from build123d import *

# Parameters (mm, degrees)
F0_W     = 1200
F0_H     = 500
F1_DEPTH = 250
F2_W     = 400
F2_H     = 260
F3_DEPTH = 250.001
F5_DEPTH = 250
F6_R     = 110
F7_DEPTH = 500.001
F8_R     = 180
F9_DEPTH = 500.001


with BuildPart() as f1:
    # F0 (on Front) → F1 (new body)
    with BuildSketch(Plane.XZ):
        Rectangle(F0_W, F0_H)
    extrude(amount=F1_DEPTH)

    # F2 (on face) → F3 (cut, through all)
    with BuildSketch(Plane(origin=(0, 0, 0), x_dir=(-1, 0, 0), z_dir=(0, 1, 0))):
        with Locations((-600, 0)):
            Rectangle(F2_W, F2_H)
        with Locations((600, 0)):
            Rectangle(F2_W, F2_H)
    extrude(amount=-F3_DEPTH, mode=Mode.SUBTRACT)

    # F4 (on face) → F5 (join)
    with BuildSketch(Plane.XZ.offset(250)):
        Polygon((0, 250), (-300, 0), (0, -250), (300, 0), align=None)
    extrude(amount=F5_DEPTH)

    # F6 (on face) → F7 (cut, through all)
    with BuildSketch(Plane.XZ.offset(500)):
        Circle(F6_R)
    extrude(amount=-F7_DEPTH, mode=Mode.SUBTRACT)

    # F8 (on face) → F9 (cut, through all)
    with BuildSketch(Plane(origin=(0, 0, -250), x_dir=(1, 0, 0), z_dir=(0, 0, -1))):
        Circle(F8_R)
    extrude(amount=-F9_DEPTH, mode=Mode.SUBTRACT)


solid = f1.part
Input: part model. Units: mm. Frame: model coordinates. A direction names the side the tool comes from. Coordinates: 2 decimals unless noted, no trailing zeros. Loops run counter-clockwise (first coordinate to the right, second up) from the corner with the lowest first, then second, coordinate; pieces in that order, holes last.
(1) Pull-direction query (Z, two-part tool) for faces 1 (the face through (362, -250, 4)), 2 (the face through (147.9, -373.25, -126.75)), 3 (the face through (501, -123, -130)); classes: released by +Z, released by -Z, zero draft, split by the parting line, or undercut.
(2) Section B-B on z = 83.5. Return the cut outline in (x, y).
(3) Section C-C on y = -327. Return the cut outline in (x, z).
(4) Material intervals for probe 1 along Z at (x, y) = (0, -380); probe 2 along X at (y, z) = (-233.5, 0); probe 3 along Z at (x, y) = (-419.5, -186), sorted ascending.
(5) First-contact query: pin 1 Ø2 at (x, z) = (-339.5, 97.5) entering from -Y; pin 2 Ø6 at (y, z) = (-402.5, 12.5) entering from +X; pin 3 Ø10 at (x, y) = (-140.5, -335) entering from +Z. Flat tips, straight axial feed; report the tip coordinate or a pass-through.
(6) Section A-A on x = -440. Return the cut outline in (y, z).
(7) Section D-D on y = -117. Return the cut outline in (x, z), then the cut area to 3 significant figures.
(8) Set-up query: faces 4 (the face through (501, -123, 130)), 5 (the face through (-152.1, -373.25, -123.25)), 6 (the face through (-499, -123, 130)). Return all of +Z, -Z, +X, -X, +Y, -Y with unobstructed straight access to the full face (end or side cutting, diameter ignored); none if empty.
Data:
1. face 1: zero draft
1. face 2: released by -Z
1. face 3: undercut
2. outline: (-400, -250) - (-199.8, -250) - (-199.8, -500) - (-71.61, -500) - (-71.61, -165.14) arc R180 cw to (-180, 0) - (-400, 0) - close; (71.61, -500) - (199.8, -500) - (199.8, -250) - (400, -250) - (400, 0) - (180, 0) arc R180 cw to (71.61, -165.14) - close
3. outline: (-300, 0) - (0, -250) - (300, 0) - (0, 250) - close; hole circle Ø220 at (0, 0)
4. probe 1: z = -250 to -110, 110 to 250
4. probe 2: x = -400 to -110, 110 to 400
4. probe 3: z = -250 to -130, 130 to 250
5. pin 1: stops at y = -250
5. pin 2: stops at x = 288.6
5. pin 3: stops at z = 137.08
6. outline: (-250, -250) - (0, -250) - (0, -130) - (-250, -130) - close; (-250, 130) - (0, 130) - (0, 250) - (-250, 250) - close
7. outline: (-600, -250) - (-136.79, -250) - (-136.79, 250) - (-600, 250) - (-600, 130) - (-400, 130) - (-400, -130) - (-600, -130) - close; (136.79, -250) - (600, -250) - (600, -130) - (400, -130) - (400, 130) - (600, 130) - (600, 250) - (136.79, 250) - close
7. area: 359,000 mm2
8. face 4: +X, +Y, -Y
8. face 5: -Z, -X, -Y
8. face 6: -X, +Y, -Y
